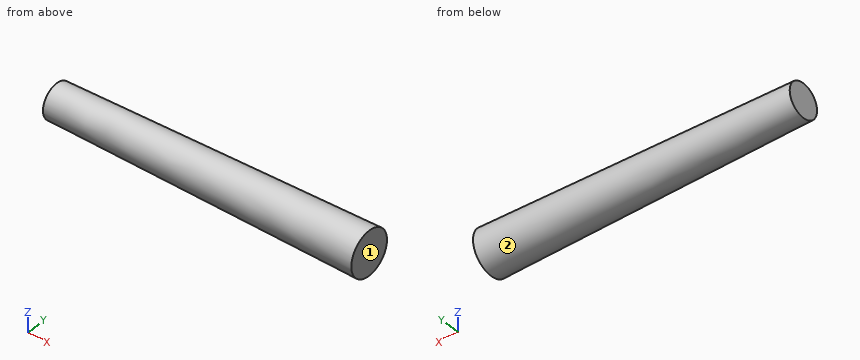
from build123d import *

# Parameters (mm, degrees)
SKIZZE4_R                       = 4.17503968
SCHNITT_LINEAR_AUSTRAGEN1_DEPTH = 5
SKIZZE7_R                       = 4.374978423
SCHNITT_LINEAR_AUSTRAGEN3_DEPTH = 5
SKIZZE8_R                       = 3.54345764
SCHNITT_LINEAR_AUSTRAGEN4_DEPTH = 5


with BuildPart() as part:
    # Skizze1 → Rotation1 (revolve)
    with BuildSketch(Plane.XY):
        Polygon((-10.538234355, 0), (-10.538234355, 2.5), (79.461765645, 4), (79.461765645, 0), align=None)
    revolve(axis=Axis((79.461765645, 0, 0), (-1, 0, 0)))

    # Skizze4 → Schnitt-Linear austragen1 (cut)
    with BuildSketch(Plane(origin=(79.461765645, 0, 0), x_dir=(0, 0, -1), z_dir=(1, 0, 0))):
        Circle(SKIZZE4_R)
    extrude(amount=-SCHNITT_LINEAR_AUSTRAGEN1_DEPTH, mode=Mode.SUBTRACT)

    # Skizze7 → Schnitt-Linear austragen3 (cut)
    with BuildSketch(Plane(origin=(74.461765645, 0, 0), x_dir=(0, 0, -1), z_dir=(1, 0, 0))):
        Circle(SKIZZE7_R)
    extrude(amount=-SCHNITT_LINEAR_AUSTRAGEN3_DEPTH, mode=Mode.SUBTRACT)

    # Skizze8 → Schnitt-Linear austragen4 (cut)
    with BuildSketch(Plane.ZY.offset(10.538234355)):
        Circle(SKIZZE8_R)
    extrude(amount=-SCHNITT_LINEAR_AUSTRAGEN4_DEPTH, mode=Mode.SUBTRACT)

    # Skizze9 → Rotation2 (revolve)
    with BuildSketch(Plane.XY):
        Polygon((69.461765645, 3.833333333), (69.461765645, 5.333333333), (-5.538234355, 4.083333333), (-5.538234355, 2.583333333), align=None)
    revolve(axis=Axis((69.461765645, 0, 0), (-1, 0, 0)))


solid = part.part
Source: CAD feature listing. Evaluate the final solid. Frame: model axes, mm. Face numbers are marked on the shaded views. A direction names the side the tool comes from. Coordinates: 2 decimals unless noted, no trailing zeros. Loops run counter-clockwise (first coordinate to the right, second up) from the corner with the lowest first, then second, coordinate; pieces in that order, holes last. Notation, with made-up numbers: (86, 19.25) - (115, 19.25) arc R17 ccw to (115, 43.25) - close; hole circle Ø6 at (-33, 70). An arc over 180 degrees is marked (long way). Return JSON: item names as keys, results as strings.
Q1. Material intervals for line 1 along Z through (x, y) = (64, 0.5); line 2 along Z through (x, y) = (60, 2.5); line 3 along Y through (x, z) = (39.5, 3.5), sorted ascending.
Results:
{"line 1": "-5.22 to 5.22", "line 2": "-4.53 to 4.53", "line 3": "-3.33 to 3.33"}
Q2. Contact query for flat-ended pins moving along their axis: P1, Ø4, axis at x = 43, z = 0.5, coming from the +Y side; P2, Ø6, axis at x = 56.5, y = -1.5, coming from the +Z side; P3, Ø3, axis at x = 57, y = -0.5, coming from the +Z side. Output: stop coordinate, or through.
Results:
{"P1": "y = 4.92", "P2": "z = 5.16", "P3": "z = 5.15"}
Q3. Access query for the marked faces 1 and 2. Directions: +Z, -Z, +X, -X, +Y, -Y. A direction counts if a zero-diameter tool reaches every point of the face in a straight line with its end or side. Return the directions, or none.
Results:
{"face 1": "+Z, -Z, +X, +Y, -Y", "face 2": "-X"}
Q4. Section B-B, the plane x = 23. Return loops of the section in (y, z).
Results:
{"outline": "circle Ø9.12 at (0, 0)"}
Q5. Section A-A, the plane x = 10.5. Return loops of the section in (y, z).
Results:
{"outline": "circle Ø8.7 at (0, 0)"}
